```python
from build123d import *

# Parameters (mm, degrees)
SKETCH1_W               = 114.3
SKETCH1_H               = 114.3
BOSS_EXTRUDE1_DEPTH     = 6.35
SKETCH2_R               = 50.8
SKETCH2_R_2             = 47.625
CUT_EXTRUDE_THIN1_DEPTH = 1.5875
SKETCH3_R               = 1.651
CUT_EXTRUDE1_DEPTH      = 3.175


with BuildPart() as part:
    # Sketch1 → Boss-Extrude1 (new body)
    with BuildSketch(Plane(origin=(0, 0, 0), x_dir=(1, 0, 0), z_dir=(0, 1, 0))):
        Rectangle(SKETCH1_W, SKETCH1_H)
    extrude(amount=BOSS_EXTRUDE1_DEPTH)

    # Sketch2 → Cut-Extrude-Thin1 (cut)
    with BuildSketch(Plane(origin=(0, 6.35, 0), x_dir=(1, 0, 0), z_dir=(0, 1, 0))):
        Circle(SKETCH2_R)
        Circle(SKETCH2_R_2, mode=Mode.SUBTRACT)
    extrude(amount=-CUT_EXTRUDE_THIN1_DEPTH, mode=Mode.SUBTRACT)

    # Sketch3 → Cut-Extrude1 (cut)
    with BuildSketch(Plane(origin=(0, 6.35, 0), x_dir=(1, 0, 0), z_dir=(0, 1, 0))):
        Circle(SKETCH3_R)
    extrude(amount=-CUT_EXTRUDE1_DEPTH, mode=Mode.SUBTRACT)


solid = part.part
```
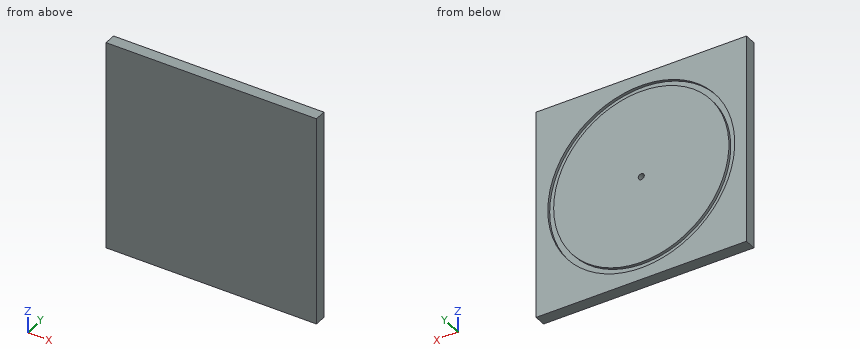
Geometry: final body of the model. Coordinates: model frame, mm. Round coordinates to 2 decimals unless told otherwise and drop trailing zeros. Order: outer loops, then holes, each group sorted by start corner. A loop starts at its lowest first (then second) coordinate and runs counter-clockwise, first axis right, second up. Notation, with made-up numbers: M 77,2.25 L 83,2.25 A26 cw 83,20.25 Z; hole C 67,-18 d9. An arc over 180 degrees is marked long. Use one line per item in the form item = value. Start each with the question number.
Q1. Material intervals for line 1 (Z direction, x = 0, y = 5.55) (3 decimals); line 2 (Z direction, x = 0, y = 3.95), sorted ascending. Write a range as [from, to].
Q2. Cut plane D-D (x = -39). Return loops of the section in (y, z).
Q3. Cut plane C-C (z = -39.5). Return loops of the section in (x, y).
Q4. Pin query (flat end, axial travel): pin 1 Ø3 at (x, z) = (0, 0) entering from +Y (3 decimals); pin 2 Ø6 at (x, z) = (4, -31) entering from -Y. Return the tip coordinate at first contact, or that it passes through.
Geometry results:
q1.line_1 = [-57.15, -50.8], [-47.625, -1.651], [1.651, 47.625], [50.8, 57.15]
q1.line_2 = [-57.15, -1.65], [1.65, 57.15]
q2.outline = M 0,-57.15 L 6.35,-57.15 L 6.35,-32.55 L 4.76,-32.55 L 4.76,-27.33 L 6.35,-27.33 L 6.35,27.33 L 4.76,27.33 L 4.76,32.55 L 6.35,32.55 L 6.35,57.15 L 0,57.15 Z
q3.outline = M -57.15,0 L 57.15,0 L 57.15,6.35 L 31.94,6.35 L 31.94,4.76 L 26.61,4.76 L 26.61,6.35 L -26.61,6.35 L -26.61,4.76 L -31.94,4.76 L -31.94,6.35 L -57.15,6.35 Z
q4.pin_1 = 3.175
q4.pin_2 = 0
